Here's how the part is built. I have some questions about the finished solid (model axes, mm). A direction names the side the tool comes from. Coordinates: 2 decimals unless noted, no trailing zeros. Order: outer loops, then holes, each group sorted by start corner. A loop starts at its lowest first (then second) coordinate and runs counter-clockwise, first axis right, second up. Notation, with made-up numbers: (48, -5) - (73, -5) arc R21 cw to (73, 3) - close; hole circle Ø11 at (-28.5, 16). An arc over 180 degrees is marked (long way). Answer as CSV lines item,"result". Start each with the question number.
Item 1: Imagine slicing it at B-B on x = 22.5. List the corners of the cut face in (y, z) for me.
Item 2: I'm going to push a flat-ended pin straight in: pin 1 (1.9 mm diameter, centred on x = -15, z = -17.5, fed in from -Y). Where does the tip first touch, or does it pass through?
Item 3: We'd pull the mould along X, two halves only. Please class faces 1 (the face through (29.287, 2.028, 14.248)), 2 (the face through (7, 4, -5)), 3 (the face through (35, 2, 0)): pulls with the +X half, pulls with the -X half, needs draft (parallel to the pull), parting line crosses it, or undercut.
Item 4: On a 3-axis mill with a long thin cutter (end or side, diameter ignored), from which of +Z, -Z, +X, -X, +Y, -Y can I reach the whole of each face in a straight line? I mean faces 4 (the face through (7, 0, -5)), 5 (the face through (-14.248, 2.028, -13.287)). Say none if no direction works.
Item 5: Imagine slicing it at A-A on z = 18.5. List the corners of the cut face in (x, y) for me.
Item 6: I need wall thicknesses on line 1 (X direction, y = 0.9, z = 18.5); line 2 (X direction, y = 2.6, z = 9); line 3 (X direction, y = 1.45, z = -17.5). Which ranges of each line are inside material? Lowest first, please.
Item 7: Imagine slicing it at D-D on x = -5. List the corners of the cut face in (y, z) for me, and give its area (3 significant figures).
Item 8: Imagine slicing it at C-C on z = -8.5. List the corners of the cut face in (x, y) for me, and give its area (3 significant figures).
from build123d import *

# Parameters (mm, degrees)
SKETCH_1_W          = 40
SKETCH_1_H          = 49
EXTRUDE_1_DEPTH     = 4
SKETCH_3_R          = 1.6
CUT_EXTRUDE_1_DEPTH = 4
SKETCH_5_W          = 15
SKETCH_5_H          = 49
SKETCH_5_R          = 2.5
EXTRUDE_2_DEPTH     = 4
CUT_EXTRUDE_2_DEPTH = 10
EXTRUDE_2_2_DEPTH   = 4
SKETCH_10_R         = 2.5
CUT_EXTRUDE_4_DEPTH = 4
FILLET_3_R          = 2.5
FILLET_4_R          = 2
SKETCH_11_R         = 2.5
CUT_EXTRUDE_5_DEPTH = 10


with BuildPart() as part:
    # 草图1 → 凸台-拉伸1 (new body)
    with BuildSketch(Plane(origin=(0, 0, 0), x_dir=(1, 0, 0), z_dir=(0, 1, 0))):
        Rectangle(SKETCH_1_W, SKETCH_1_H)
    extrude(amount=EXTRUDE_1_DEPTH)

    # 草图3 → 切除-拉伸1 (cut)
    with BuildSketch(Plane(origin=(0, 4, 0), x_dir=(1, 0, 0), z_dir=(0, 1, 0))):
        with Locations(Location((-5, -18.5, 0), (0, 0, 270))):
            Circle(SKETCH_3_R)
        with Locations(Location((15, -18.5, 0), (0, 0, 270))):
            Circle(SKETCH_3_R)
        with Locations(Location((-15, 17.5, 0), (0, 0, 270))):
            Circle(SKETCH_3_R)
        with Locations(Location((5, 17.5, 0), (0, 0, 270))):
            Circle(SKETCH_3_R)
    extrude(amount=-CUT_EXTRUDE_1_DEPTH, mode=Mode.SUBTRACT)

    # 草图5 → Extrude 2 (add)
    with BuildSketch(Plane.XZ):
        with Locations((27.5, 0)):
            Rectangle(SKETCH_5_W, SKETCH_5_H)
        with Locations(Location((27.5, -15.781639971, 0), (0, 0, 270))):
            Circle(SKETCH_5_R, mode=Mode.SUBTRACT)
    extrude(amount=-EXTRUDE_2_DEPTH)

    # 草图6 → 切除-拉伸2 (cut)
    with BuildSketch(Plane.XZ):
        with BuildLine():
            Line((30, 15), (-15, 15))
            Line((-15, 15), (-15, -14))
            Line((-15, -14), (18.168560721, -14))
            ThreePointArc((18.168560721, -14), (22.470467132, -7.722247989), (30, -6.616488581))
            Line((30, -6.616488581), (30, 15))
        make_face()
    extrude(amount=-CUT_EXTRUDE_2_DEPTH, mode=Mode.SUBTRACT)

    # 草图8 → Extrude 2 2 (add)
    with BuildSketch(Plane.XZ):
        Polygon((-18.101802033, -1.000622031), (-16.101802033, -1.790346265), (35.304944651, -22.088923087), (9.496940315, 16.662915832), (8.164977494, 18.662915832), (3.171096865, 15.337084168), (4.503059685, 13.337084168), (19.695055349, -9.474356855), (-13.898197967, 3.790346265), (-15.898197967, 4.580070499), align=None)
    extrude(amount=-EXTRUDE_2_2_DEPTH)

    # 草图10 → 切除-拉伸4 (cut)
    with BuildSketch(Plane.XZ):
        with Locations(Location((27.5, -15.781639971, 0), (0, 0, 270))):
            Circle(SKETCH_10_R)
        Polygon((35.304944651, -22.088923087), (35, -21.968511997), (35, -21.631035455), align=None)
    extrude(amount=-CUT_EXTRUDE_4_DEPTH, mode=Mode.SUBTRACT)

    # 圆角3
    fillet_3_edges = [part.edges().sort_by_distance(p)[0] for p in [
        (30, 2, -6.616488581),
        (-15, 2, -14),
        (-15, 2, 15),
        (30, 2, 15),
        (3.395588654, 2, 15),
        (10.604411346, 2, 15),
        (-15, 2, 4.225406148),
        (-15, 2, -2.225406148),
        (14.819507483, 2, -14),
        (25.000500065, 2, -6.616352192),
        (19.695055349, 2, -9.474356855),
    ]]
    fillet(fillet_3_edges, radius=FILLET_3_R)

    # 圆角4
    fillet_4_edges = [part.edges().sort_by_distance(p)[0] for p in [
        (35, 2, 24.5),
        (35, 2, -24.5),
        (-20, 2, 24.5),
        (-20, 2, -24.5),
    ]]
    fillet(fillet_4_edges, radius=FILLET_4_R)

    # 草图11 → 切除-拉伸5 (cut)
    with BuildSketch(Plane.XZ):
        with Locations(Location((17.5, -15.781639971, 0), (0, 0, 270))):
            Circle(SKETCH_11_R)
    extrude(amount=-CUT_EXTRUDE_5_DEPTH, mode=Mode.SUBTRACT)


solid = part.part
Responses:
1,outline,"(0, -24.5) - (4, -24.5) - (4, -2.86) - (0, -2.86) - close; (0, 15) - (4, 15) - (4, 24.5) - (0, 24.5) - close"
2,pin 1,"passes through"
3,face 1,"undercut"
3,face 2,"needs draft"
3,face 3,"pulls with the +X half"
4,face 4,"+Z, -Z, +X, -X, -Y"
4,face 5,"+Y, -Y"
5,outline,"(-20, 0) - (-6.6, 0) - (-6.6, 4) - (-20, 4) - close; (-3.4, 0) - (13.4, 0) - (13.4, 4) - (-3.4, 4) - close; (16.6, 0) - (35, 0) - (35, 4) - (16.6, 4) - close"
6,line 1,"x = -20 to -6.6, -3.4 to 13.4, 16.6 to 35"
6,line 2,"x = -20 to -15, 7.39 to 14.6, 30 to 35"
6,line 3,"x = -20 to -16.6, -13.4 to 3.4, 6.6 to 15.68, 19.32 to 25.68, 29.32 to 35"
7,outline,"(0, -24.5) - (4, -24.5) - (4, -14) - (0, -14) - close; (0, -6.17) - (4, -6.17) - (4, 0.28) - (0, 0.28) - close; (0, 15) - (4, 15) - (4, 16.9) - (0, 16.9) - close; (0, 20.1) - (4, 20.1) - (4, 24.5) - (0, 24.5) - close"
7,area,"93.0 mm^2"
8,outline,"(-20, 0) - (-15, 0) - (-15, 4) - (-20, 4) - close; (0.89, 0) - (35, 0) - (35, 4) - (0.89, 4) - close"
8,area,"156 mm^2"
